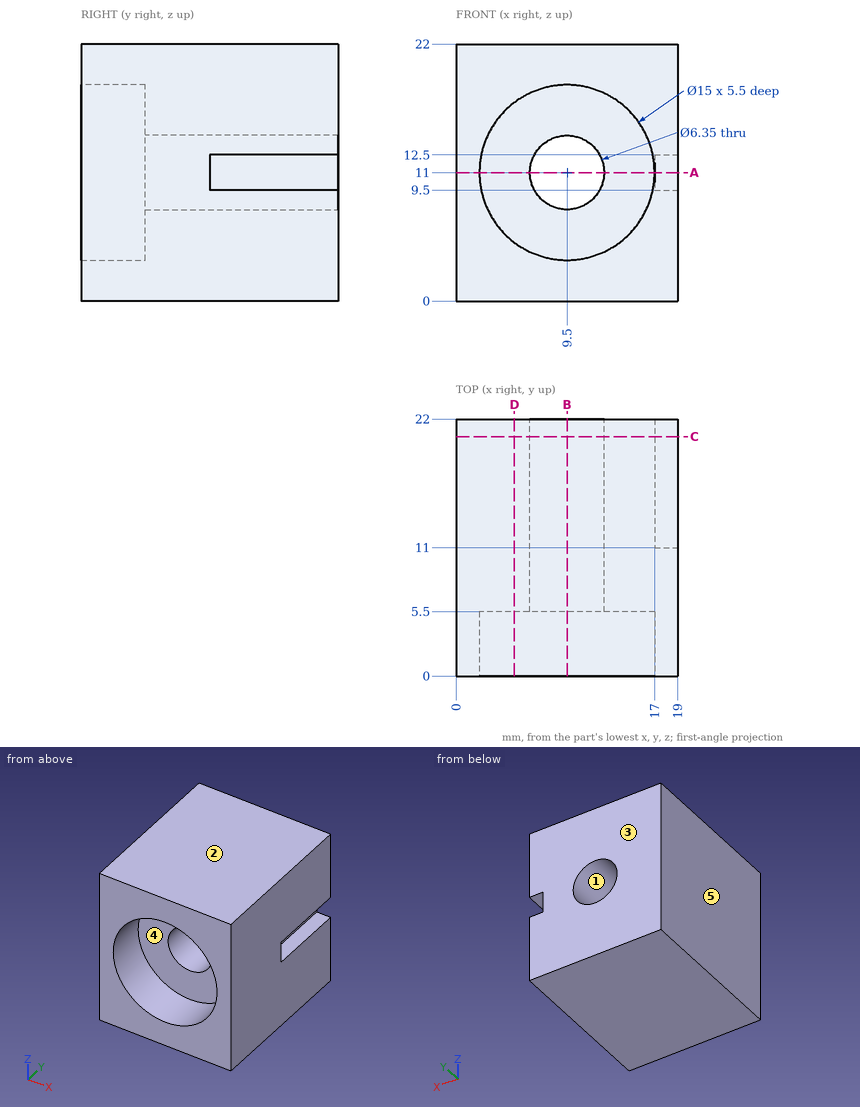
The figure shows three views and two pictorial views of one solid part (mm, origin at its lowest corner). Answer the questions. A direction names the side the tool comes from. Give positions to 0.01 mm unless a question says otherwise; leave off trailing zeros. Write each loop counter-clockwise with the first axis right and the second up, starting at its lowest first coordinate (ties: lowest second). Pieces come first, ordered by that corner, then holes. Notation, with made-up numbers: (52.5, -19.75) - (93.5, -19.75) arc R20 ccw to (93.5, -3.75) - close; hole circle Ø11 at (77.25, 43.25). An arc over 180 degrees is marked (long way). Use one line per item in the form item = value.
1. A cutting plane is placed at B-B (x = 9.5). Write down the section's boundary in (y, z) (3 decimals).
Filled in:
outline = (0, 0) - (22, 0) - (22, 7.825) - (5.5, 7.825) - (5.5, 3.5) - (0, 3.5) - close; (0, 18.5) - (5.5, 18.5) - (5.5, 14.175) - (22, 14.175) - (22, 22) - (0, 22) - close
2. For the marked faces 4 and 5, determine the directions among +Z, -Z, +X, -X, +Y, -Y from which every point of the face is accessible in a straight line to the end or side of a thin tool.
Filled in:
face_4 = -Y
face_5 = +Z, -Z, -X, +Y, -Y
3. Determine the mould class of the marked faces 1, 2 and 3 for opening direction Z: released by +Z, released by -Z, zero draft, split by the parting line, or undercut.
Filled in:
face_1 = undercut
face_2 = released by +Z
face_3 = zero draft
4. A cutting plane is placed at A-A (z = 11). Write down the section's boundary in (x, y) (3 decimals).
Filled in:
outline = (0, 0) - (2, 0) - (2, 5.5) - (6.325, 5.5) - (6.325, 22) - (0, 22) - close; (12.675, 5.5) - (17, 5.5) - (17, 0) - (19, 0) - (19, 11) - (17, 11) - (17, 22) - (12.675, 22) - close
5. A cutting plane is placed at D-D (x = 5). Write down the section's boundary in (y, z).
Filled in:
outline = (0, 0) - (22, 0) - (22, 22) - (0, 22) - (0, 17) - (5.5, 17) - (5.5, 5) - (0, 5) - close
6. Consider L1, parallel to X at y = 15.25, z = 11 (3 decimals); L2, parallel to X at y = 2, z = 11; L3, parallel to Y at x = 12.25, z = 14.5. Determine where each line is inside the solid, lowest interval first.
Filled in:
L1 = 0 to 6.325, 12.675 to 17
L2 = 0 to 2, 17 to 19
L3 = 5.5 to 22
7. A cutting plane is placed at C-C (y = 20.5). Write down the section's boundary in (x, z) (3 decimals).
Filled in:
outline = (0, 0) - (19, 0) - (19, 9.5) - (17, 9.5) - (17, 12.5) - (19, 12.5) - (19, 22) - (0, 22) - close; hole circle Ø6.35 at (9.5, 11)
8. Each of these flat-tipped pins is pushed along its axis until it touches: pin 1 Ø1 at (x, z) = (7, 11) entering from -Y; pin 2 Ø7.5 at (x, z) = (10.5, 9.5) entering from -Y. Where does it stop, or does it pass through?
Filled in:
pin_1 = through
pin_2 = 5.5
